from build123d import *

# Parameters (mm, degrees)
SKETCH1_W                      = 127.660000204
SKETCH1_H                      = 31.75
BOSS_EXTRUDE1_DEPTH            = 6.35
M5X0_8_TAPPED_HOLE1_AT_2_COUNT = 2
M5X0_8_TAPPED_HOLE1_AT_2_PITCH = 19.05
F_16_0MM_DOWEL_HOLE1_D         = 16
TAP_DRILL_FOR_M4X0_7_TAP1_D    = 3.3


with BuildPart() as part:
    # Sketch1 → Boss-Extrude1 (new, symmetric)
    with BuildSketch(Plane(origin=(0, 0, 0), x_dir=(1, 0, 0), z_dir=(0, 1, 0))):
        Rectangle(SKETCH1_W, SKETCH1_H)
    extrude(amount=BOSS_EXTRUDE1_DEPTH, both=True)

    # Sketch4 → M5x0.8 Tapped Hole1 (revolve, cut)
    with BuildSketch(Plane(origin=(-63.830000102, 0, 9.525), x_dir=(0, 0, 1), z_dir=(0, 1, 0))):
        Polygon((0, 0), (0, 12.192), (2.1, 10.9301927), (2.1, 0), align=None)
    m5x0_8_tapped_hole1 = revolve(axis=Axis((-70.180000102, 0, 9.525), (1, 0, 0)), mode=Mode.SUBTRACT)

    # M5x0.8 Tapped Hole1 at 2: M5x0.8 Tapped Hole1 ×2
    with Locations(*[(0, 0, -i * M5X0_8_TAPPED_HOLE1_AT_2_PITCH) for i in range(1, M5X0_8_TAPPED_HOLE1_AT_2_COUNT)]):
        add(m5x0_8_tapped_hole1, mode=Mode.SUBTRACT)

    # Mirror1: M5x0.8 Tapped Hole1 across plane
    add(m5x0_8_tapped_hole1.mirror(Plane(origin=(0, 0, 0), x_dir=(0, 0, 1), z_dir=(1, 0, 0))), mode=Mode.SUBTRACT)

    # Mirror1 copy 1 sketch → Mirror1 copy 1 (revolve, cut)
    with BuildSketch(Plane(origin=(63.830000102, 0, -9.525), x_dir=(0, 0, 1), z_dir=(0, 1, 0))):
        Polygon((0, 0), (0, -12.192), (2.1, -10.9301927), (2.1, 0), align=None)
    revolve(axis=Axis((70.180000102, 0, -9.525), (1, 0, 0)), mode=Mode.SUBTRACT)

    # Ø16.0mm Dowel Hole1 (through all)
    with Locations(Plane(origin=(0, 6.35, 0), x_dir=(1, 0, 0), z_dir=(0, 1, 0))):
        with Locations((0, 0)):
            Hole(F_16_0MM_DOWEL_HOLE1_D / 2)

    # Tap Drill for M4x0.7 Tap1 (through all)
    with Locations(Plane(origin=(0, 6.35, 0), x_dir=(1, 0, 0), z_dir=(0, 1, 0))):
        with Locations((0, 12), (12, 0), (-12, 0), (0, -12)):
            Hole(TAP_DRILL_FOR_M4X0_7_TAP1_D / 2)


solid = part.part
Model file for the job. Use its own axes, mm. A direction names the side the tool comes from. Give positions to 0.01 mm unless a question says otherwise; leave off trailing zeros. Loops run counter-clockwise (first coordinate to the right, second up) from the corner with the lowest first, then second, coordinate; pieces in that order, holes last.
1) Pull direction Z, two halves, no side cores. Call faces 1 (the flat face through (-1, 0, 15.875)), 2 (the flat face through (-63.83, 0, 0)), 3 (the cylindrical face through (10.476, -0.089, 0.632)), 4 (the cylindrical face through (-58.441, -0.092, 7.427)): +Z half, -Z half, draft (parallel to the pull), parting line (faces both ways), or undercut.
2) Wall check: line 1 (Z direction, x = 61, y = 0) (3 decimals); line 2 (Z direction, x = 0, y = -1) (3 decimals); line 3 (Z direction, x = 12, y = 0.25) (3 decimals). Give the ranges that are in metal, low to high.
3) Saw through at A-A (x = 12). Write the cut outline in (y, z) (3 decimals), plus the area to 3 significant figures.
4) Saw through at B-B (y = -4.5). Write the cut outline in (x, z) (3 decimals), plus the area to 3 significant figures.
5) Flat gauge pins, fed straight in: pin 1 Ø2.5 at (y, z) = (0, -9.525) entering from -X; pin 2 Ø2 at (x, z) = (0, 12) entering from +Y; pin 3 Ø2.5 at (y, z) = (0, 9.525) entering from +X. Where does each tip first touch, or does it go through?
6) Saw through at D-D (x = -11.5). Write the cut outline in (y, z) (3 decimals).
7) Tool access for faces 5 (the cylindrical face through (58.44, -2.08, -9.8)), 6 (the cylindrical face through (-58.44, -2.08, -9.8)), 7 (the cylindrical face through (0.4, -0.1, -10.4)): list every direction of +Z, -Z, +X, -X, +Y, -Y with a clear straight run to the whole face (end or side of a thin tool).
8) Saw through at C-C (z = 0). Write the cut outline in (x, y).
Answer block:
1. face 1: +Z half
1. face 2: draft
1. face 3: undercut
1. face 4: undercut
2. line 1: z = -15.875 to -11.625, -7.425 to 7.425, 11.625 to 15.875
2. line 2: z = -15.875 to -13.65, -10.35 to -8, 8 to 10.35, 13.65 to 15.875
2. line 3: z = -15.875 to -1.65, 1.65 to 15.875
3. outline: (-6.35, -15.875) - (6.35, -15.875) - (6.35, -1.65) - (-6.35, -1.65) - close; (-6.35, 1.65) - (6.35, 1.65) - (6.35, 15.875) - (-6.35, 15.875) - close
3. area: 361 mm2
4. outline: (-63.83, -15.875) - (63.83, -15.875) - (63.83, 15.875) - (-63.83, 15.875) - close; hole circle Ø3.3 at (-12, 0); hole circle Ø16 at (0, 0); hole circle Ø3.3 at (0, -12); hole circle Ø3.3 at (0, 12); hole circle Ø3.3 at (12, 0)
4. area: 3,820 mm2
5. pin 1: stops at x = -52.39
5. pin 2: passes through
5. pin 3: stops at x = 52.39
6. outline: (-6.35, -15.875) - (6.35, -15.875) - (6.35, -1.572) - (-6.35, -1.572) - close; (-6.35, 1.572) - (6.35, 1.572) - (6.35, 15.875) - (-6.35, 15.875) - close
7. face 5: +X
7. face 6: -X
7. face 7: +Y, -Y
8. outline: (-63.83, -6.35) - (-13.65, -6.35) - (-13.65, 6.35) - (-63.83, 6.35) - close; (-10.35, -6.35) - (-8, -6.35) - (-8, 6.35) - (-10.35, 6.35) - close; (8, -6.35) - (10.35, -6.35) - (10.35, 6.35) - (8, 6.35) - close; (13.65, -6.35) - (63.83, -6.35) - (63.83, 6.35) - (13.65, 6.35) - close
